Could you check a few things on this model? Use its own coordinates, in mm. A direction names the side the tool comes from. Round coordinates to 2 decimals unless told otherwise and drop trailing zeros. Loops run counter-clockwise (first coordinate to the right, second up) from the corner with the lowest first, then second, coordinate; pieces in that order, holes last. Notation, with made-up numbers: M 10,-37 L 19,-37 A26 ccw 19,-6 Z; hole C 45.5,-1.75 d5. An arc over 180 degrees is marked long. One line per item, written item: value. Start each with the question number.
Q1. Imagine slicing it at C-C (z = 2.4). Please give me the cut outline in (x, y).
Q2. Thinking about a two-plate mould opening in X: for faces 1 (the face through (2.192, -4.214, 1.838)), 2 (the face through (11.923, 3.755, 0.887)), 3 (the face through (-7.35, 7.35, 2)), which applies, released by +X, released by -X, zero draft, split by the parting line, or undercut?
Q3. Imagine slicing it at A-A (y = 0). Please give me the cut outline in (x, z).
Q4. Which directions (+Z, -Z, +X, -X, +Y, -Y) give clear straight access to the entire face, cutting with the end or side of a thin tool? Please do faces 4 (the face through (-2.17, -9.76, 1.41)), 5 (the face through (3, -3, 0)).
Q5. Please list where these lines run through material, in increasing order: line 1 along Z through (x, y) = (-11.25, -3); line 2 along Z through (x, y) = (-4.25, -3.75); line 3 along Y through (x, z) = (-8, 1.2).
Q6. I'm going to push flat-ended pins straight in: pin 1 Ø12 at (x, y) = (8.5, 10) entering from +Z; pin 2 Ø1.8 at (x, y) = (0, 0) entering from -Z; pin 3 Ø1 at (x, z) = (5, 0.5) entering from +Y; pin 4 Ø1.5 at (x, z) = (-3.5, 1.5) entering from +Y. Where does each tip first touch, or does it pass through?
from build123d import *

# Parameters (mm, degrees)
F0_R     = 12.5
F1_DEPTH = 2
F2_R     = 10
F3_DEPTH = 1
F4_R     = 4.75
F5_DEPTH = 1.7
F6_R     = 1.5
F7_DEPTH = 25
F8_SIZE  = 1.8
F9_R     = 0.2


with BuildPart() as f1:
    # F0 (on Top) → F1 (new body)
    with BuildSketch(Plane.XY):
        Circle(F0_R)
    extrude(amount=F1_DEPTH)

    # F2 (on face) → F3 (cut)
    with BuildSketch(Plane.XY.offset(2)):
        Circle(F2_R)
    extrude(amount=-F3_DEPTH, mode=Mode.SUBTRACT)

    # F4 (on face) → F5 (join)
    with BuildSketch(Plane.XY.offset(1)):
        Circle(F4_R)
    extrude(amount=F5_DEPTH)

    # F6 (on face) → F7 (cut)
    with BuildSketch(Plane.XY.offset(2.7)):
        Circle(F6_R)
    extrude(amount=-F7_DEPTH, mode=Mode.SUBTRACT)

    # F8
    f8_edges = [f1.edges().sort_by_distance(p)[0] for p in [
        (-1.5, 0, 0),
    ]]
    chamfer(f8_edges, length=F8_SIZE)

    # F9
    f9_edges = [f1.edges().sort_by_distance(p)[0] for p in [
        (-12.5, 0, 2),
        (-10, 0, 2),
    ]]
    fillet(f9_edges, radius=F9_R)


solid = f1.part
Report:
1. outline: C 0,0 d9.5; hole C 0,0 d3
2. face 1: undercut
2. face 2: split by the parting line
2. face 3: zero draft
3. outline: M -12.5,0 L -3.3,0 L -1.5,1.8 L -1.5,2.7 L -4.75,2.7 L -4.75,1 L -10,1 L -10,1.8 A0.2 ccw -10.2,2 L -12.3,2 A0.2 ccw -12.5,1.8 Z; M 1.5,1.8 L 3.3,0 L 12.5,0 L 12.5,1.8 A0.2 ccw 12.3,2 L 10.2,2 A0.2 ccw 10,1.8 L 10,1 L 4.75,1 L 4.75,2.7 L 1.5,2.7 Z
4. face 4: +Z
4. face 5: -Z, +X, -X, +Y, -Y
5. line 1: z = 0 to 2
5. line 2: z = 0 to 1
5. line 3: y = -9.6 to -6, 6 to 9.6
6. pin 1: stops at z = 2
6. pin 2: passes through
6. pin 3: stops at y = 11.66
6. pin 4: stops at y = 12.19
